```python
from build123d import *

# Parameters (mm, degrees)
SKETCH1_R               = 6.5
BOSS_EXTRUDE1_DEPTH     = 10
SKETCH2_OUTSIDE_W       = 38.674
SKETCH2_OUTSIDE_H       = 35.58
SKETCH2_OUTSIDE_R       = 10
CUT_EXTRUDE1_DEPTH      = 3
CUT_EXTRUDE1_DRAFT      = -50
MIRROR1_COPY_1_SKETCH_W = 38.674
MIRROR1_COPY_1_SKETCH_H = 35.58
MIRROR1_COPY_1_SKETCH_R = 10
MIRROR1_COPY_1_DEPTH    = 3
MIRROR1_COPY_1_DRAFT    = -50
CHAMFER1_SIZE           = 0.3


with BuildPart() as part:
    # Sketch1 → Boss-Extrude1 (new body)
    with BuildSketch(Plane.XY):
        Polygon((-11.547005384, 0), (-5.773502692, -10), (5.773502692, -10), (11.547005384, 0), (5.773502692, 10), (-5.773502692, 10), align=None)
        Circle(SKETCH1_R, mode=Mode.SUBTRACT)
    extrude(amount=BOSS_EXTRUDE1_DEPTH)


with BuildPart() as cut_extrude1_tool:
    # Sketch2 outside → Cut-Extrude1 (with draft: the straight prism first)
    with BuildSketch(Plane.XY.offset(10)):
        Rectangle(SKETCH2_OUTSIDE_W, SKETCH2_OUTSIDE_H)
        Circle(SKETCH2_OUTSIDE_R, mode=Mode.SUBTRACT)
    extrude(amount=-CUT_EXTRUDE1_DEPTH)
    # Cut-Extrude1: the draft: its side faces are tilted about the plane it starts from
    cut_extrude1_sides = [cut_extrude1_tool.faces().sort_by_distance(p)[0] for p in [
        (0, -17.79, 8.5),
        (19.337, 0, 8.5),
        (0, 17.79, 8.5),
        (-19.337, 0, 8.5),
        (-10, 0, 8.5),
    ]]
    draft(cut_extrude1_sides, Plane.XY.offset(10), CUT_EXTRUDE1_DRAFT)


with BuildPart() as part_1:
    add(part.part)

    # Cut-Extrude1: cut by cut_extrude1_tool
    add(cut_extrude1_tool.part, mode=Mode.SUBTRACT)


with BuildPart() as mirror1_copy_1_tool:
    # Mirror1 copy 1 sketch → Mirror1 copy 1 (with draft: the straight prism first)
    with BuildSketch(Plane(origin=(0, 0, 0), x_dir=(1, 0, 0), z_dir=(0, 0, -1))):
        Rectangle(MIRROR1_COPY_1_SKETCH_W, MIRROR1_COPY_1_SKETCH_H)
        Circle(MIRROR1_COPY_1_SKETCH_R, mode=Mode.SUBTRACT)
    extrude(amount=-MIRROR1_COPY_1_DEPTH)
    # Mirror1 copy 1: the draft: its side faces are tilted about the plane it starts from
    mirror1_copy_1_sides = [mirror1_copy_1_tool.faces().sort_by_distance(p)[0] for p in [
        (0, -17.79, 1.5),
        (19.337, 0, 1.5),
        (0, 17.79, 1.5),
        (-19.337, 0, 1.5),
        (-10, 0, 1.5),
    ]]
    draft(mirror1_copy_1_sides, Plane(origin=(0, 0, 0), x_dir=(1, 0, 0), z_dir=(0, 0, -1)), MIRROR1_COPY_1_DRAFT)


with BuildPart() as part_2:
    add(part_1.part)

    # Mirror1 copy 1: cut by mirror1_copy_1_tool
    add(mirror1_copy_1_tool.part, mode=Mode.SUBTRACT)

    # Chamfer1
    chamfer1_edges = [part_2.edges().sort_by_distance(p)[0] for p in [
        (-6.5, 0, 0),
        (-6.5, 0, 10),
    ]]
    chamfer(chamfer1_edges, length=CHAMFER1_SIZE)


solid = part_2.part
```
Check sheet for the modelled part. Datum: model origin and axes. Units: mm. Coordinates: 2 decimals unless noted, no trailing zeros. Loops run counter-clockwise (first coordinate to the right, second up) from the corner with the lowest first, then second, coordinate; pieces in that order, holes last.
1) Gauge pin test, flat ends, axial feed: pin 1 (1 mm diameter, centred on y = 6, z = 1, fed in from -X); pin 2 (3 mm diameter, centred on y = 6.5, z = 7.5, fed in from -X); pin 3 (3 mm diameter, centred on y = 3.5, z = 4.5, fed in from +X); pin 4 (5 mm diameter, centred on x = 0, y = -7.5, fed in from -Z). Record the tip position at first contact, or that the pin passes through.
2) Material ranges on probe 1 along X at (y, z) = (2, 9.75); probe 2 along X at (y, z) = (5.5, 6.25); probe 3 along Y at (x, z) = (-4.25, 3.25), recorded low to high.
3) Sectioned sample at A-A (z = 1.75). Record the boundary of the cut face in (x, y).
4) Release check for a two-part mould opening along Y. For faces 1 (the face through (7, -2, 10)), 2 (the face through (5.206, -8.967, 0.309)), 3 (the face through (-5.158, -3.955, 4.934)) record: released by +Y, released by -Y, zero draft, split by the parting line, or undercut.
Check sheet entries:
1. pin 1: stops at x = -8.37
1. pin 2: stops at x = -8.66
1. pin 3: stops at x = 10.39
1. pin 4: stops at z = 0
2. probe 1: x = -10.1 to -6.24, 6.24 to 10.1
2. probe 2: x = -8.37 to -3.46, 3.46 to 8.37
2. probe 3: y = -10 to -4.92, 4.92 to 10
3. outline: (-11.55, 0) - (-5.77, -10) - (5.77, -10) - (11.55, 0) - (5.77, 10) - (-5.77, 10) - close; hole circle Ø13 at (0, 0)
4. face 1: zero draft
4. face 2: released by -Y
4. face 3: undercut
